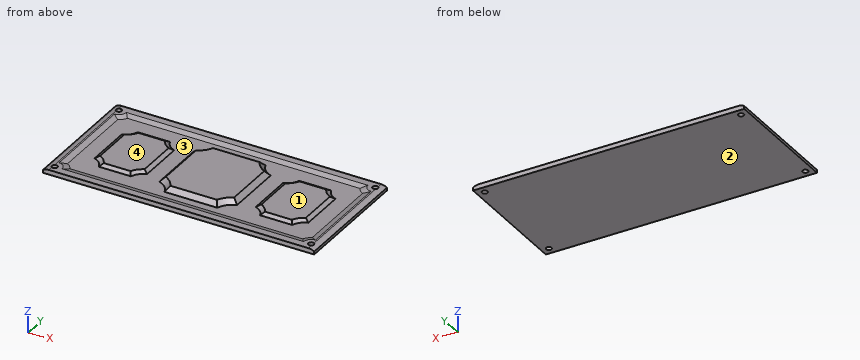
from build123d import *

# Parameters (mm, degrees)
SKETCH2_W           = 174.5
SKETCH2_H           = 80
BOSS_EXTRUDE1_DEPTH = 3
SKETCH3_R           = 1.75
CUT_EXTRUDE1_DEPTH  = 3
CUT_EXTRUDE2_DEPTH  = 1
CUT_EXTRUDE2_DRAFT  = -75
CUT_EXTRUDE3_REACH  = 120.413
BOSS_EXTRUDE2_DEPTH = 3
BOSS_EXTRUDE2_TAPER = 45
BOSS_EXTRUDE3_DEPTH = 1.5
BOSS_EXTRUDE3_TAPER = 60


# Read off the part's stored shape, not the designer's step: Cut-Extrude2
with BuildPart() as part:
    # Sketch2 → Boss-Extrude1 (new body)
    with BuildSketch(Plane.XY):
        Rectangle(SKETCH2_W, SKETCH2_H)
    extrude(amount=BOSS_EXTRUDE1_DEPTH)

    # Sketch3 → Cut-Extrude1 (cut)
    with BuildSketch(Plane.XY.offset(3)):
        with Locations((-82.5, 35.25)):
            Circle(SKETCH3_R)
        with Locations((82.5, 35.25)):
            Circle(SKETCH3_R)
        with Locations((82.5, -35.25)):
            Circle(SKETCH3_R)
        with Locations((-82.5, -35.25)):
            Circle(SKETCH3_R)
    extrude(amount=-CUT_EXTRUDE1_DEPTH, mode=Mode.SUBTRACT)


with BuildPart() as cut_extrude2_tool:
    # Cut-Extrude2 outline → Cut-Extrude2 (with draft: the straight prism first)
    with BuildSketch(Plane.XY.offset(2)):
        with BuildLine():
            ThreePointArc((-74.883112009, 31.517949192), (-76.502284356, 29.252284356), (-78.767949192, 27.633112009))
            Line((-78.767949192, 27.633112009), (-78.767949192, -27.633112009))
            ThreePointArc((-78.767949192, -27.633112009), (-76.502284356, -29.252284356), (-74.883112009, -31.517949192))
            Line((-74.883112009, -31.517949192), (74.883112009, -31.517949192))
            ThreePointArc((74.883112009, -31.517949192), (76.502284356, -29.252284356), (78.767949192, -27.633112009))
            Line((78.767949192, -27.633112009), (78.767949192, 27.633112009))
            ThreePointArc((78.767949192, 27.633112009), (76.502284356, 29.252284356), (74.883112009, 31.517949192))
            Line((74.883112009, 31.517949192), (-74.883112009, 31.517949192))
        make_face()
    extrude(amount=CUT_EXTRUDE2_DEPTH)
    # Cut-Extrude2: the draft: its side faces are tilted about the plane it starts from
    cut_extrude2_sides = [cut_extrude2_tool.faces().sort_by_distance(p)[0] for p in [
        (-76.502284356, 29.252284356, 2.5),
        (-78.767949192, 0, 2.5),
        (-76.502284356, -29.252284356, 2.5),
        (0, -31.517949192, 2.5),
        (76.502284356, -29.252284356, 2.5),
        (78.767949192, 0, 2.5),
        (76.502284356, 29.252284356, 2.5),
        (0, 31.517949192, 2.5),
    ]]
    draft(cut_extrude2_sides, Plane.XY.offset(2), CUT_EXTRUDE2_DRAFT)


with BuildPart() as part_1:
    add(part.part)

    # Cut-Extrude2: cut by cut_extrude2_tool
    add(cut_extrude2_tool.part, mode=Mode.SUBTRACT)

    # Sketch5 → Cut-Extrude3 (cut, up to next)
    with BuildSketch(Plane(origin=(0, 40, 0), x_dir=(1, 0, 0), z_dir=(0, 1, 0)), mode=Mode.PRIVATE) as cut_extrude3_sk1:
        with BuildLine():
            Line((-87.25, -1.910795209), (-87.25, -3))
            Line((-87.25, -3), (-83.5, -3))
            ThreePointArc((-83.5, -3), (-85.45248989, -2.722185897), (-87.25, -1.910795209))
        make_face()
    cut_extrude3_tool1 = extrude(cut_extrude3_sk1.sketch, amount=-CUT_EXTRUDE3_REACH, mode=Mode.PRIVATE) & part_1.part
    cut_extrude3 = cut_extrude3_tool1.solids().sort_by_distance((-86.327713, 40, 2.678112))[0]
    add(cut_extrude3, mode=Mode.SUBTRACT)

    # Mirror1: Cut-Extrude3 across plane
    add(cut_extrude3.mirror(Plane(origin=(0, 0, 0), x_dir=(0, 0, 1), z_dir=(1, 0, 0))), mode=Mode.SUBTRACT)

    # Sketch6 → Boss-Extrude2 (add)
    with BuildSketch(Plane.XY.offset(2)):
        with BuildLine():
            Line((-25, 18.539708909), (-25, -18.539708909))
            ThreePointArc((-25, -18.539708909), (-20.014718626, -21.532667818), (-17.021759717, -26.517949192))
            Line((-17.021759717, -26.517949192), (17.021759717, -26.517949192))
            ThreePointArc((17.021759717, -26.517949192), (20.014718626, -21.532667818), (25, -18.539708909))
            Line((25, -18.539708909), (25, 18.539708909))
            ThreePointArc((25, 18.539708909), (20.014718626, 21.532667818), (17.021759717, 26.517949192))
            Line((17.021759717, 26.517949192), (-17.021759717, 26.517949192))
            ThreePointArc((-17.021759717, 26.517949192), (-20.014718626, 21.532667818), (-25, 18.539708909))
        make_face()
    extrude(amount=BOSS_EXTRUDE2_DEPTH, taper=BOSS_EXTRUDE2_TAPER)

    # Sketch7 → Boss-Extrude3 (add)
    with BuildSketch(Plane.XY.offset(2)):
        with BuildLine():
            ThreePointArc((-68.767949192, -14.978557178), (-64.696881381, -17.446881381), (-62.228557178, -21.517949192))
            Line((-62.228557178, -21.517949192), (-41.539392014, -21.517949192))
            ThreePointArc((-41.539392014, -21.517949192), (-39.071067812, -17.446881381), (-35, -14.978557178))
            Line((-35, -14.978557178), (-35, 14.978557178))
            ThreePointArc((-35, 14.978557178), (-39.071067812, 17.446881381), (-41.539392014, 21.517949192))
            Line((-41.539392014, 21.517949192), (-62.228557178, 21.517949192))
            ThreePointArc((-62.228557178, 21.517949192), (-64.696881381, 17.446881381), (-68.767949192, 14.978557178))
            Line((-68.767949192, 14.978557178), (-68.767949192, -14.978557178))
        make_face()
    boss_extrude3 = extrude(amount=BOSS_EXTRUDE3_DEPTH, taper=BOSS_EXTRUDE3_TAPER)

    # Mirror2: Boss-Extrude3 across plane
    add(boss_extrude3.mirror(Plane(origin=(0, 0, 0), x_dir=(0, 0, 1), z_dir=(1, 0, 0))))


solid = part_1.part
For this review, take the finished solid that the model builds, in its own axes (mm). Face numbers are marked on the shaded views. A direction names the side the tool comes from. Round coordinates to 2 decimals unless told otherwise and drop trailing zeros. Order: outer loops, then holes, each group sorted by start corner. A loop starts at its lowest first (then second) coordinate and runs counter-clockwise, first axis right, second up. Notation, with made-up numbers: M -36,-16.75 L -30,-16.75 A20 ccw -30,-7.75 Z; hole C -17,71.5 d11. An arc over 180 degrees is marked long. Use a Markdown table: item, result. Add a question column.
Item 1: Tool access review of the marked faces 1, 2, 3 and 4: name each direction out of +Z, -Z, +X, -X, +Y, -Y from which nothing blocks a thin tool from reaching the whole face with its end or side.
Item 2: Insertion check: pin 1 (14.5 mm diameter, centred on x = -57.5, y = 8, fed in from +Z); pin 2 (4 mm diameter, centred on x = -38, y = -23.5, fed in from +Z); pin 3 (2 mm diameter, centred on x = -40.5, y = 20.5, fed in from +Z). Each pin has a flat end and moves straight along its axis. Give the tip position at first contact, or say it passes through.
Item 3: To check wall thickness, follow line 1 along Y through (x, z) = (-82.5, 1); line 2 along X through (y, z) = (35.25, 1); line 3 along Z through (x, y) = (-70.5, 26.5). State the ranges of each line that lie inside material, in increasing order.
Item 4: Add section A-A, the plane y = -0.5. Give the boundary of the cut face in (x, z), then the cut area to 3 significant figures.
Item 5: Add section B-B, the plane x = 3.5. Give the boundary of the cut face in (y, z).
Geometry results:
| question | item | result |
|---|---|---|
| 1 | face 1 | +Z, +X, +Y, -Y |
| 1 | face 2 | -Z, +X, -X, +Y, -Y |
| 1 | face 3 | +Z |
| 1 | face 4 | +Z, -X, +Y, -Y |
| 2 | pin 1 | stops at z = 3.5 |
| 2 | pin 2 | stops at z = 2 |
| 2 | pin 3 | stops at z = 2.23 |
| 3 | line 1 | y = -40 to -37, -33.5 to 33.5, 37 to 40 |
| 3 | line 2 | x = -87.25 to -84.25, -80.75 to 80.75, 84.25 to 87.25 |
| 3 | line 3 | z = 0 to 2 |
| 4 | outline | M -87.25,0 L 87.25,0 L 87.25,1.91 A7 ccw 83.5,3 L 82.5,3 L 78.77,2 L 68.77,2 L 66.17,3.5 L 37.6,3.5 L 35,2 L 25,2 L 22,5 L -22,5 L -25,2 L -35,2 L -37.6,3.5 L -66.17,3.5 L -68.77,2 L -78.77,2 L -82.5,3 L -83.5,3 A7 ccw -87.25,1.91 Z |
| 4 | area | 594 mm² |
| 5 | outline | M -40,0 L 40,0 L 40,3 L 35.25,3 L 31.52,2 L 26.52,2 L 23.52,5 L -23.52,5 L -26.52,2 L -31.52,2 L -35.25,3 L -40,3 Z |
